The model under review builds one solid part; all positions refer to its coordinate system, in mm. A direction names the side the tool comes from. Round coordinates to 2 decimals unless told otherwise and drop trailing zeros. Order: outer loops, then holes, each group sorted by start corner. A loop starts at its lowest first (then second) coordinate and runs counter-clockwise, first axis right, second up. Notation, with made-up numbers: (-26.5, 66) -> (30.5, 66) arc R10 ccw to (30.5, 85) -> close; hole circle Ø9 at (31, -29). An arc over 180 degrees is marked (long way). Use a Markdown table: item, result. Add a question column.
```python
from build123d import *

# Parameters (mm, degrees)
F0_W     = 39.9
F0_H     = 5.9
F1_DEPTH = 5
F3_DEPTH = 3
F4_R     = 1.1
F5_DEPTH = 13


with BuildPart() as f1:
    # F0 (on Top) → F1 (new body)
    with BuildSketch(Plane.XY):
        Rectangle(F0_W, F0_H)
    extrude(amount=F1_DEPTH)

    # F2 (on Front) → F3 (join, symmetric)
    with BuildSketch(Plane.XZ):
        with BuildLine():
            Line((-19.95, 5), (19.95, 5))
            ThreePointArc((19.95, 5), (0, 24.95), (-19.95, 5))
        make_face()
    extrude(amount=F3_DEPTH, both=True)

    # F4 (on face) → F5 (cut)
    with BuildSketch(Plane(origin=(0, 0, 0), x_dir=(1, 0, 0), z_dir=(0, 0, -1))):
        with Locations((15, 0)):
            Circle(F4_R)
        with Locations((-15, 0)):
            Circle(F4_R)
    extrude(amount=-F5_DEPTH, mode=Mode.SUBTRACT)


solid = f1.part
```
Q1. For faces 5 (the face through (-15, 0, 13)), 6 (the face through (0, 3, 13)), 7 (the face through (0, -2.95, 2)), list the 3-axis set-ups (+Z, -Z, +X, -X, +Y, -Y) from which the entire face can be reached by the end or side of a thin tool; tool diameter is ignored.
Q2. For pin 1 (1.5 mm diameter, centred on x = -6.5, z = 1.5, fed in from -Y); pin 2 (1.5 mm diameter, centred on x = -9, z = 2.5, fed in from +Y); pin 3 (1.8 mm diameter, centred on x = 15, y = 0, fed in from -Z), all flat-tipped, find the tip position at first contact; note any pin that passes through.
Q3. Draft analysis for pull direction X (two halves, no side actions). For faces 1 (the face through (0, 2.95, 2)), 2 (the face through (19.95, 0, 2)), 3 (the face through (13.9, 0, 6.4)), 4 (the face through (-19.95, 0, 2)), state which applies: released by +X, released by -X, zero draft, split by the parting line, or undercut.
Q4. Add section B-B, the plane y = -0.5. Give the boundary of the cut face in (x, z).
Q5. Add section D-D, the plane x = 15. Give the boundary of the cut face in (y, z), then the cut area to 3 significant figures.
Q6. To check wall thickness, follow line 1 along Y through (x, z) = (15, 3.75); line 2 along X through (y, z) = (0, 9); line 3 along X through (y, z) = (-0.75, 11.25). State the ranges of each line that lie inside material, in increasing order.
Q7. Add section A-A, the plane x = 6. Give the boundary of the cut face in (y, z).
Q8. Add section C-C, the plane z = 5.5. Give the boundary of the cut face in (x, y).
Return value:
| question | item | result |
|---|---|---|
| 1 | face 5 | -Z |
| 1 | face 6 | +Z, -Z, +X, -X, +Y |
| 1 | face 7 | -Z, +X, -X, -Y |
| 2 | pin 1 | y = -2.95 |
| 2 | pin 2 | y = 2.95 |
| 2 | pin 3 | z = 13 |
| 3 | face 1 | zero draft |
| 3 | face 2 | released by +X |
| 3 | face 3 | undercut |
| 3 | face 4 | released by -X |
| 4 | outline | (-19.95, 0) -> (-15.98, 0) -> (-15.98, 13) -> (-14.02, 13) -> (-14.02, 0) -> (14.02, 0) -> (14.02, 13) -> (15.98, 13) -> (15.98, 0) -> (19.95, 0) -> (19.95, 5) arc R19.95 ccw to (-19.95, 5) -> close |
| 5 | outline | (-3, 5) -> (-2.95, 5) -> (-2.95, 0) -> (-1.1, 0) -> (-1.1, 13) -> (1.1, 13) -> (1.1, 0) -> (2.95, 0) -> (2.95, 5) -> (3, 5) -> (3, 18.15) -> (-3, 18.15) -> close |
| 5 | area | 79.8 mm² |
| 6 | line 1 | -2.95 to -1.1, 1.1 to 2.95 |
| 6 | line 2 | -19.54 to -16.1, -13.9 to 13.9, 16.1 to 19.54 |
| 6 | line 3 | -18.95 to -15.8, -14.2 to 14.2, 15.8 to 18.95 |
| 7 | outline | (-3, 5) -> (-2.95, 5) -> (-2.95, 0) -> (2.95, 0) -> (2.95, 5) -> (3, 5) -> (3, 24.03) -> (-3, 24.03) -> close |
| 8 | outline | (-19.94, -3) -> (19.94, -3) -> (19.94, 3) -> (-19.94, 3) -> close; hole circle Ø2.2 at (-15, 0); hole circle Ø2.2 at (15, 0) |
